```python
from build123d import *

# Parameters (mm, degrees)
CROQUIS1_R              = 12.5
SALIENTE_EXTRUIR1_DEPTH = 10
SALIENTE_EXTRUIR2_DEPTH = 12
CROQUIS3_R              = 2.25
CORTAR_EXTRUIR1_DEPTH   = 66.117202028
CROQUIS4_R              = 4.25
CORTAR_EXTRUIR2_DEPTH   = 66.117202081


with BuildPart() as part:
    # Croquis1 → Saliente-Extruir1 (new body)
    with BuildSketch(Plane(origin=(0, 0, 0), x_dir=(0, 0, -1), z_dir=(1, 0, 0))):
        Circle(CROQUIS1_R)
        with BuildLine():
            Line((-1.658312395, -2.5), (1.658312395, -2.5))
            ThreePointArc((1.658312395, -2.5), (0, 3), (-1.658312395, -2.5))
        make_face(mode=Mode.SUBTRACT)
    extrude(amount=SALIENTE_EXTRUIR1_DEPTH)

    # Croquis2 → Saliente-Extruir2 (add)
    with BuildSketch(Plane(origin=(10, 0, 0), x_dir=(0, 0, -1), z_dir=(1, 0, 0))):
        with BuildLine():
            Line((-9.987492178, 50.5), (-12.484365222, 0.625))
            ThreePointArc((-12.484365222, 0.625), (0, -12.5), (12.484365222, 0.625))
            Line((12.484365222, 0.625), (9.987492178, 50.5))
            ThreePointArc((9.987492178, 50.5), (0, 60), (-9.987492178, 50.5))
        make_face()
    extrude(amount=SALIENTE_EXTRUIR2_DEPTH)

    # Croquis3 → Cortar-Extruir1 (cut, through all)
    with BuildSketch(Plane(origin=(0, 0, 0), x_dir=(1, 0, 0), z_dir=(0, 1, 0))):
        with Locations(Location((5, 0, 0), (0, 0, 227.478835592))):
            Circle(CROQUIS3_R)
    extrude(amount=-CORTAR_EXTRUIR1_DEPTH, mode=Mode.SUBTRACT)

    # Croquis4 → Cortar-Extruir2 (cut, through all)
    with BuildSketch(Plane(origin=(22, 0, 0), x_dir=(0, 0, -1), z_dir=(1, 0, 0))):
        with Locations((0, 50)):
            Circle(CROQUIS4_R)
    extrude(amount=-CORTAR_EXTRUIR2_DEPTH, mode=Mode.SUBTRACT)


solid = part.part
```
The listing builds one solid part. Answer for the finished solid, in the listing's coordinates (mm). A direction names the side the tool comes from. Round coordinates to 2 decimals unless told otherwise and drop trailing zeros. Loops run counter-clockwise (first coordinate to the right, second up) from the corner with the lowest first, then second, coordinate; pieces in that order, holes last.
Q1. For a pull along Z with two mould halves and no side action, classify faces 4 (the face through (22, 24, 0)), 5 (the face through (16.08, 45.85, 0.92)), 6 (the face through (16, 60, 0)) as released by +Z, released by -Z, zero draft, split by the parting line, or undercut.
Q2. Section C-C, the plane y = 47.5 is taken. Determine the outline of the cut face in (x, z).
Q3. Section D-D, the plane z = 7 is taken. Determine the outline of the cut face in (x, y).
Q4. Section A-A, the plane z = 0 is taken. Determine the outline of the cut face in (x, y), then the cut area to 3 significant figures.
Q5. Given pin 1 Ø10 at (x, z) = (10.5, 9) entering from +Y; pin 2 Ø1.7 at (x, z) = (2, 0) entering from +Y; pin 3 Ø1 at (y, z) = (24, 5) entering from -X, each flat-ended and moving along its own axis, determine where each tip first touches the part or whether it passes through.
Q6. Which of the six approach directions +Z, -Z, +X, -X, +Y, -Y give full straight-line access (tool end or side, diameter ignored) to faces 1 (the face through (2.96, -7.17, 0.95)), 2 (the face through (9, -2.5, 0)), 3 (the face through (0, -3, 0))?
Q7. Find the intervals of material crossed by line 1 (Z direction, x = 2.75, y = 0); line 2 (X direction, y = -9.25, z = 0); line 3 (X direction, y = 23, z = -6.75), in increasing order.
Completed:
1. face 4: zero draft
1. face 5: undercut
1. face 6: split by the parting line
2. outline: (10, -10.14) - (22, -10.14) - (22, -3.44) - (10, -3.44) - close; (10, 3.44) - (22, 3.44) - (22, 10.14) - (10, 10.14) - close
3. outline: (0, -10.36) - (22, -10.36) - (22, 57.14) - (10, 57.14) - (10, 10.36) - (0, 10.36) - close
4. outline: (0, -12.5) - (2.75, -12.5) - (2.75, -2.5) - (0, -2.5) - close; (0, 3) - (10, 3) - (10, -2.5) - (7.25, -2.5) - (7.25, -12.5) - (22, -12.5) - (22, 45.75) - (10, 45.75) - (10, 12.5) - (0, 12.5) - close; (10, 54.25) - (22, 54.25) - (22, 60) - (10, 60) - close
4. area: 918 mm2
5. pin 1: stops at y = 59.17
5. pin 2: stops at y = 12.5
5. pin 3: stops at x = 10
6. face 1: -Y
6. face 2: -X
6. face 3: +Z, -Z, -X, +Y, -Y
7. line 1: z = -12.5 to -3, 3 to 12.5
7. line 2: x = 0 to 2.75, 7.25 to 22
7. line 3: x = 10 to 22
